Model file for the job. Use its own axes, mm. Face numbers are marked on the shaded views. A direction names the side the tool comes from. Coordinates: 2 decimals unless noted, no trailing zeros. Loops run counter-clockwise (first coordinate to the right, second up) from the corner with the lowest first, then second, coordinate; pieces in that order, holes last. Notation, with made-up numbers: (64.5, -23) -> (109.5, -23) arc R25 ccw to (109.5, 8) -> close; hole circle Ø11 at (80.5, 63). An arc over 180 degrees is marked (long way). Use one line per item in the form item = value.
```python
from build123d import *

# Parameters (mm, degrees)
BOSS_EXTRUDE1_DEPTH                              = 49
SKETCH2_W                                        = 45
SKETCH2_H                                        = 2
BOSS_EXTRUDE2_DEPTH                              = 4
SKETCH3_W                                        = 45
SKETCH3_H                                        = 2
BOSS_EXTRUDE3_DEPTH                              = 4
SKETCH4_W                                        = 45
SKETCH4_H                                        = 36
CUT_EXTRUDE1_DEPTH                               = 16.5
CUT_EXTRUDE2_REACH                               = 51
SKETCH5_W                                        = 28
SKETCH5_H                                        = 15.499999955
SKETCH6_W                                        = 28
SKETCH6_H                                        = 15.499999989
CUT_EXTRUDE3_DEPTH                               = 50
CUT_EXTRUDE4_DEPTH                               = 34.052463428
CBORE_FOR_M2_HEX_HEAD_MACHINE_SCREW1_AT_COUNT    = 2
CBORE_FOR_M2_HEX_HEAD_MACHINE_SCREW1_AT_PITCH    = 32
CBORE_FOR_M2_HEX_HEAD_MACHINE_SCREW2_D           = 2.5
CBORE_FOR_M2_HEX_HEAD_MACHINE_SCREW2_DEPTH       = 15.445359267
CBORE_FOR_M2_HEX_HEAD_MACHINE_SCREW2_CBORE_D     = 5
CBORE_FOR_M2_HEX_HEAD_MACHINE_SCREW2_CBORE_DEPTH = 3.850389414
F_3_4_3_4_DIAMETER_HOLE1_D                       = 3.4
F_3_4_3_4_DIAMETER_HOLE1_DEPTH                   = 2
F_2_4_2_4_DIAMETER_HOLE1_D                       = 2.4
F_2_4_2_4_DIAMETER_HOLE1_DEPTH                   = 2
F_3_4_3_4_DIAMETER_HOLE2_D                       = 3.4
F_3_4_3_4_DIAMETER_HOLE2_DEPTH                   = 40
F_2_4_2_4_DIAMETER_HOLE2_D                       = 2.4
F_2_4_2_4_DIAMETER_HOLE2_DEPTH                   = 40
FILLET1_R                                        = 2


with BuildPart() as part:
    # Sketch1 → Boss-Extrude1 (new body)
    with BuildSketch(Plane(origin=(24.5, 0, 0), x_dir=(0, 0, -1), z_dir=(1, 0, 0))):
        Polygon((20, 18.5), (-20, 18.5), (-20, 0), (-20.001723757, -0.999998514), (17.070392977, -10.933442255), (20, 0), align=None)
    extrude(amount=-BOSS_EXTRUDE1_DEPTH)

    # Sketch2 → Boss-Extrude2 (add)
    with BuildSketch(Plane(origin=(0, 18.5, 0), x_dir=(-1, 0, 0), z_dir=(0, 1, 0))):
        with Locations((0, 19)):
            Rectangle(SKETCH2_W, SKETCH2_H)
    extrude(amount=BOSS_EXTRUDE2_DEPTH)

    # Sketch3 → Boss-Extrude3 (add)
    with BuildSketch(Plane(origin=(0, 18.5, 0), x_dir=(-1, 0, 0), z_dir=(0, 1, 0))):
        with Locations((0, -19)):
            Rectangle(SKETCH3_W, SKETCH3_H)
    extrude(amount=BOSS_EXTRUDE3_DEPTH)

    # Sketch4 → Cut-Extrude1 (cut)
    with BuildSketch(Plane(origin=(0, 18.5, 0), x_dir=(-1, 0, 0), z_dir=(0, 1, 0))):
        Rectangle(SKETCH4_W, SKETCH4_H)
    extrude(amount=-CUT_EXTRUDE1_DEPTH, mode=Mode.SUBTRACT)

    # Sketch5 → Cut-Extrude2 (cut, up to next)
    with BuildSketch(Plane(origin=(24.5, 0, 0), x_dir=(0, 0, -1), z_dir=(1, 0, 0)), mode=Mode.PRIVATE) as cut_extrude2_sk1:
        with Locations((0, 10.750000023)):
            Rectangle(SKETCH5_W, SKETCH5_H)
    cut_extrude2_tool1 = extrude(cut_extrude2_sk1.sketch, amount=-CUT_EXTRUDE2_REACH, mode=Mode.PRIVATE) & part.part
    add(cut_extrude2_tool1.solids().sort_by_distance((24.5, 10.75, 0))[0], mode=Mode.SUBTRACT)

    # Sketch6 → Cut-Extrude3 (cut, through all)
    with BuildSketch(Plane.ZY.offset(24.5)):
        with Locations((0, 10.750000006)):
            Rectangle(SKETCH6_W, SKETCH6_H)
    extrude(amount=-CUT_EXTRUDE3_DEPTH, mode=Mode.SUBTRACT)

    # Sketch7 → Cut-Extrude4 (cut, through all)
    with BuildSketch(Plane(origin=(0, -5.933442255, 1.589861061), x_dir=(1, 0, 0), z_dir=(0, -0.965925826, 0.258819045))):
        with BuildLine():
            Line((-9, -8.75), (-9, -13.75))
            Line((-9, -13.75), (9, -13.75))
            Line((9, -13.75), (9, -10.71870086))
            ThreePointArc((9, -10.71870086), (9.500097813, -9.395714303), (10.750293429, -8.73435043))
            ThreePointArc((10.750293429, -8.73435043), (11.989102808, -8.085784512), (12.500293429, -6.784258263))
            ThreePointArc((12.500293429, -6.784258263), (13.097950879, -5.392242266), (14.5, -4.818516526))
            Line((14.5, -4.818516526), (20.5, -4.818516526))
            Line((20.5, -4.818516526), (20.5, 4.818516526))
            Line((20.5, 4.818516526), (14.499827541, 4.818516526))
            ThreePointArc((14.499827541, 4.818516526), (13.092195397, 5.397752032), (12.499913771, 6.79994478))
            ThreePointArc((12.499913771, 6.79994478), (11.993841738, 8.11119891), (10.75, 8.765686517))
            ThreePointArc((10.75, 8.765686517), (9.5, 9.427124344), (9, 10.75))
            Line((9, 10.75), (9, 13.75))
            Line((9, 13.75), (-9, 13.75))
            Line((-9, 13.75), (-9, 10.71870086))
            ThreePointArc((-9, 10.71870086), (-9.500097813, 9.395714303), (-10.750293429, 8.73435043))
            ThreePointArc((-10.750293429, 8.73435043), (-11.989102808, 8.085784512), (-12.500293429, 6.784258263))
            ThreePointArc((-12.500293429, 6.784258263), (-13.097950879, 5.392242266), (-14.5, 4.818516526))
            Line((-14.5, 4.818516526), (-20.5, 4.818516526))
            Line((-20.5, 4.818516526), (-20.5, -4.818516526))
            Line((-20.5, -4.818516526), (-12.5, -4.818516526))
            Line((-12.5, -4.818516526), (-12.5, -8.75))
            Line((-12.5, -8.75), (-9, -8.75))
        make_face()
    extrude(amount=-CUT_EXTRUDE4_DEPTH, mode=Mode.SUBTRACT)

    # Sketch8 → CBORE for M2 Hex Head Machine Screw1 (revolve, cut)
    with BuildSketch(Plane(origin=(-16, 2.647047613, -11.767559682), x_dir=(0, 0.258819045, 0.965925826), z_dir=(1, 0, 0))):
        Polygon((0, 0), (0, 21.3402415), (1.25, 21.3402415), (1.25, 9.745271647), (2.5, 9.745271647), (2.5, 0), align=None)
    cbore_for_m2_hex_head_machine_screw1 = revolve(axis=Axis((-16, 8.78067661, -13.411060619), (0, -0.965925826, 0.258819045)), mode=Mode.SUBTRACT)

    # CBORE for M2 Hex Head Machine Screw1 at: CBORE for M2 Hex Head Machine Screw1 ×2
    with Locations(*[(i * CBORE_FOR_M2_HEX_HEAD_MACHINE_SCREW1_AT_PITCH, 0, 0) for i in range(1, CBORE_FOR_M2_HEX_HEAD_MACHINE_SCREW1_AT_COUNT)]):
        add(cbore_for_m2_hex_head_machine_screw1, mode=Mode.SUBTRACT)

    # CBORE for M2 Hex Head Machine Screw2
    with Locations(Plane(origin=(0, -0.282400026, 0.075668859), x_dir=(1, 0, 0), z_dir=(0, 0.965925826, -0.258819045))):
        with Locations((-16, -11.318516526), (16, -11.318516526)):
            CounterBoreHole(CBORE_FOR_M2_HEX_HEAD_MACHINE_SCREW2_D / 2, CBORE_FOR_M2_HEX_HEAD_MACHINE_SCREW2_CBORE_D / 2, CBORE_FOR_M2_HEX_HEAD_MACHINE_SCREW2_CBORE_DEPTH, depth=CBORE_FOR_M2_HEX_HEAD_MACHINE_SCREW2_DEPTH)

    # Ø3.4 (3.4) Diameter Hole1
    with Locations(Plane.XY.offset(-18)):
        with Locations((15, 6.1), (-15, 6.1), (15, 20.1), (-15, 20.1)):
            Hole(F_3_4_3_4_DIAMETER_HOLE1_D / 2, depth=F_3_4_3_4_DIAMETER_HOLE1_DEPTH)

    # Ø2.4 (2.4) Diameter Hole1
    with Locations(Plane.XY.offset(-18)):
        with Locations((-11, 19.1), (-11, 7.1), (11, 19.1), (11, 7.1)):
            Hole(F_2_4_2_4_DIAMETER_HOLE1_D / 2, depth=F_2_4_2_4_DIAMETER_HOLE1_DEPTH)

    # Ø3.4 (3.4) Diameter Hole2
    with Locations(Plane.XY.offset(20)):
        with Locations((15, 6.1), (-15, 6.1), (15, 20.1), (-15, 20.1)):
            Hole(F_3_4_3_4_DIAMETER_HOLE2_D / 2, depth=F_3_4_3_4_DIAMETER_HOLE2_DEPTH)

    # Ø2.4 (2.4) Diameter Hole2
    with Locations(Plane.XY.offset(20)):
        with Locations((-11, 19.1), (-11, 7.1), (11, 19.1), (11, 7.1)):
            Hole(F_2_4_2_4_DIAMETER_HOLE2_D / 2, depth=F_2_4_2_4_DIAMETER_HOLE2_DEPTH)

    # Fillet1
    fillet1_edges = [part.edges().sort_by_distance(p)[0] for p in [
        (-9, -3.09905445, -8.228277441),
        (-12.5, -2.590283051, -4.294431133),
        (-20.5, -2.590283051, -4.294431133),
        (-20.5, -1.343159204, 5.348393808),
        (-9, -0.187340192, 14.285245134),
        (9, -0.187340192, 14.285245134),
        (20.5, -1.343159204, 5.348393808),
        (20.5, -2.590283051, -4.294431133),
        (9, -3.746102063, -13.231282458),
        (-9, -3.746102063, -13.231282458),
    ]]
    fillet(fillet1_edges, radius=FILLET1_R)


solid = part.part
```
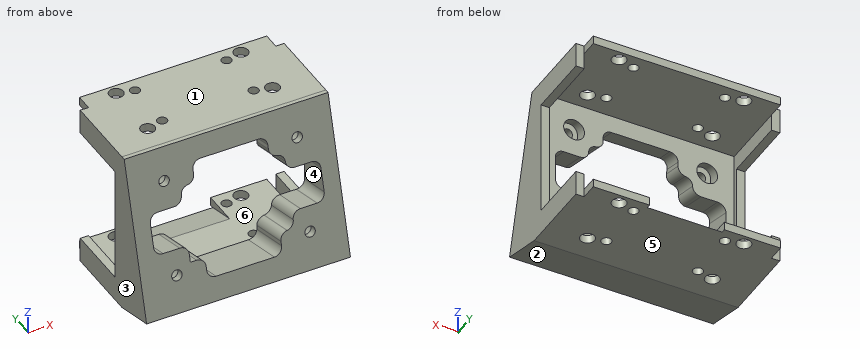
Q1. Band-saw the part on A-A, the plane y = 12.5. Write the cut outline in (x, z).
Result:
outline = (-24.5, -20) -> (24.5, -20) -> (24.5, -14) -> (22.5, -14) -> (22.5, -18) -> (-22.5, -18) -> (-22.5, -14) -> (-24.5, -14) -> close; (-24.5, 14) -> (-22.5, 14) -> (-22.5, 18) -> (22.5, 18) -> (22.5, 14) -> (24.5, 14) -> (24.5, 20) -> (-24.5, 20) -> close
Q2. Wall check: line 1 along Z through (x, y) = (-20, 13); line 2 along X through (y, z) = (19, 19); line 3 along X through (y, z) = (10.5, 16). Give the ranges that are in metal, low to high.
Result:
line_1 = -20 to -18, 18 to 20
line_2 = -22.5 to -16.3, -13.7 to -12.2, -9.8 to 9.8, 12.2 to 13.7, 16.3 to 22.5
line_3 = -24.5 to -22.5, 22.5 to 24.5
Q3. Which spindle directions (+Z, -Z, +X, -X, +Y, -Y) get a long thin tool onto all of the face, cutting with end or side? Do the marked faces 5 and 6. Say none if no direction does.
Result:
face_5 = -Z, +X, -X, +Y, -Y
face_6 = +Y
Q4. Band-saw the part on D-D, the plane z = 15.5. Write the cut outline in (x, y), and give its area (3 significant figures).
Result:
outline = (-24.5, -2.21) -> (24.5, -2.21) -> (24.5, 18.5) -> (22.5, 18.5) -> (22.5, 2) -> (-22.5, 2) -> (-22.5, 18.5) -> (-24.5, 18.5) -> close
area = 272 mm2
Q5. Mould opens along Z. For the marked faces 1, 2, 3 and 4 say: released by +Z, released by -Z, zero draft, split by the parting line, or undercut.
Result:
face_1 = released by +Z
face_2 = released by -Z
face_3 = zero draft
face_4 = undercut
Q6. Band-saw the part on C-C, the plane z = 0.5. Write the cut outline in (x, y), and give its area (3 significant figures).
Result:
outline = (-24.5, -6.23) -> (-20.5, -6.23) -> (-20.5, 2) -> (-22.5, 2) -> (-22.5, 3) -> (-24.5, 3) -> close; (20.5, -6.23) -> (24.5, -6.23) -> (24.5, 3) -> (22.5, 3) -> (22.5, 2) -> (20.5, 2) -> close
area = 69.8 mm2
Q7. Pin check, flat tips, straight feed: pin 1 Ø1.6 at (x, z) = (23, 6) entering from +Y; pin 2 Ø2 at (x, y) = (11, 7.1) entering from -Z. Stop position of each tip, or through.
Result:
pin_1 = 3
pin_2 = through
Q8. Band-saw the part on B-B, the plane x = 2. Write the cut outline in (y, z).
Result:
outline = (-10.93, -17.07) -> (0, -20) -> (21.52, -20) -> (14.05, -18) -> (2, -18) -> (2, -14.77) -> (-9.49, -11.69) -> close; (-2.37, 14.87) -> (2, 13.7) -> (2, 18) -> (22.5, 18) -> (22.5, 20) -> (0, 20) -> (-1, 20) -> close
